Part model, mm, in its own coordinate system. A direction names the side the tool comes from. Round coordinates to 2 decimals unless told otherwise and drop trailing zeros. Write each loop counter-clockwise with the first axis right and the second up, starting at its lowest first coordinate (ties: lowest second). Pieces come first, ordered by that corner, then holes. Notation, with made-up numbers: (83, 84) -> (113, 84) arc R16 cw to (113, 102) -> close; hole circle Ø9 at (-30, 4). An arc over 180 degrees is marked (long way). Use CSV: the item, a comma, the result in double quotes. Start each with the question number.
Autodesk Inventor part; units mm, degrees
ref_plane "YZ Plane" through (0, 0, 0) normal (1, 0, 0) x (0, 1, 0)
ref_plane "XZ Plane" through (0, 0, 0) normal (0, 1, 0) x (-1, 0, 0)
ref_plane "XY Plane" through (0, 0, 0) normal (0, 0, 1) x (1, 0, 0)
sketch "Sketch1" plane through (0, 0, 0) normal (0, 1, 0) x (-1, 0, 0)
  line L0 (0, 0) -> (40, 0)
  line L1 (40, 0) -> (40, -40)
  line L2 (40, -40) -> (0, -40)
  line L3 (0, -40) -> (0, 0)
  dimension "d0" = 40
  dimension "d1" = 40
extrude "Extrusion1" add sketch "Sketch1" along normal blind 5
sketch "Sketch2" plane through (0, 5, 0) normal (0, 1, 0) x (1, 0, 0)
  circle A0 centre (-20, 20) radius 17.5
  point P0 (0, 0)
  dimension "d4" = 35
ref_plane "Work Plane1" through (0, 25, 0) normal (0, 1, 0) x (1, 0, 0)
sketch "Sketch3" plane through (0, 25, 0) normal (0, 1, 0) x (1, 0, 0)
  circle A0 centre (-20, 20) radius 11
  point P0 (0, 0)
  dimension "d6" = 22
loft "Loft1" add profiles "Sketch2", "Sketch3"
sketch "Sketch6" plane through (0, 25, 0) normal (0, 1, 0) x (1, 0, 0)
  circle A0 centre (-20, 20) radius 9
  circle A1 centre (-20, 20) radius 11
  point P0 (0, 0)
  dimension "d15" = 18
sketch "Sketch8" plane through (0, 0, 0) normal (0, -1, 0) x (1, 0, 0)
  circle A0 centre (-20, -20) radius 16.5
  point P0 (0, 0)
  dimension "d16" = 33
loft "Loft2" cut profiles "Sketch8", "Sketch6" contours all / A0
sketch "Sketch9" plane through (0, 25, 0) normal (0, 1, 0) x (1, 0, 0)
  circle A0 centre (-20, 20) radius 11
  circle A1 centre (-20, 20) radius 9
  point P0 (0, 0)
  dimension "d21" = 22
  dimension "d22" = 18
extrude "Extrusion3" add sketch "Sketch9" along normal blind 10
hole "Hole1" at (-36, 5, -4) direction (0, -1, 0) diameter 3.5 end through all
hole "Hole2" at (-4, 5, -4) direction (0, -1, 0) diameter 3.5 end through all
hole "Hole3" at (-4, 5, -36) direction (0, -1, 0) diameter 3.5 end through all
hole "Hole4" at (-36, 5, -36) direction (0, -1, 0) diameter 3.5 end through all
properties part number "FanAdapter"
1. Drill centre lines: line 1 along X through (y, z) = (4, -4); line 2 along Z through (x, y) = (-20, 28). Where is each one in solid material? Low to high. Write a range as [from, to].
2. Band-saw the part on B-B (y = 21). List the corners of the cut face in (x, z), then the cut area to 3 significant figures.
3. Which spindle directions (+Z, -Z, +X, -X, +Y, -Y) get a long thin tool onto all of the face, cutting with end or side? Do faces 1 (the flat face through (0, 2, -20)), 2 (the cylindrical face through (-14.924, 29.93, -29.759)). Say none if no direction does.
4. Pull direction X, two halves, no side cores. Call faces 3 (the flat face through (-40, 2, -20)), 4 (the flat face through (-20, 2, -40)), 5 (the cylindrical face through (-34.29, 2.46, -36.38)), 6 (the conical face through (-28.82, 15.1, -11.91)): released by +X, released by -X, zero draft, split by the parting line, or undercut.
5. Flat gauge pins, fed straight in: pin 1 (12 mm diameter, centred on x = -11.5, y = 17.5, fed in from +Z); pin 2 (10 mm diameter, centred on x = -6.5, y = 12, fed in from +Z); pin 3 (2 mm diameter, centred on x = -35.5, y = 18, fed in from +Z); pin 4 (5.5 mm diameter, centred on x = -4, z = -36, fed in from +Y). Where does each tip first touch, or does it go through?
6. Band-saw the part on A-A (x = -20). List the corners of the cut face in (y, z).
Answers below:
1,line 1,"x = [-40, -37.75], [-34.25, -5.75], [-2.25, 0]"
1,line 2,"z = [-31, -29], [-11, -9]"
2,outline,"circle Ø24.6 at (-20, -20); hole circle Ø20.4 at (-20, -20)"
2,area,"148 mm^2"
3,face 1,"+Z, -Z, +X, +Y, -Y"
3,face 2,"+Y"
4,face 3,"released by -X"
4,face 4,"zero draft"
4,face 5,"undercut"
4,face 6,"undercut"
5,pin 1,"stops at z = -5.8"
5,pin 2,"stops at z = -6.84"
5,pin 3,"passes through"
5,pin 4,"stops at y = 5"
6,outline,"(0, -40) -> (5, -40) -> (5, -37.5) -> (25, -31) -> (35, -31) -> (35, -29) -> (25, -29) -> (0, -36.5) -> close; (0, -3.5) -> (25, -11) -> (35, -11) -> (35, -9) -> (25, -9) -> (5, -2.5) -> (5, 0) -> (0, 0) -> close"
